from build123d import *

# Parameters (mm, degrees)
F0_R     = 11.5
F2_DEPTH = 2.3
F1_R     = 1.55
F3_DEPTH = 25
F4_R     = 1
F5_R     = 0.2


with BuildPart() as f2:
    # F0 (on Top) → F2 (new body)
    with BuildSketch(Plane.XY):
        Circle(F0_R)
    extrude(amount=F2_DEPTH)

    # F1 (on Top) → F3 (cut)
    with BuildSketch(Plane.XY):
        with Locations((0, -8.5)):
            Circle(F1_R)
    extrude(amount=F3_DEPTH, mode=Mode.SUBTRACT)

    # F4
    f4_edges = [f2.edges().sort_by_distance(p)[0] for p in [
        (-11.5, 0, 2.3),
        (-11.5, 0, 0),
    ]]
    fillet(f4_edges, radius=F4_R)

    # F5
    f5_edges = [f2.edges().sort_by_distance(p)[0] for p in [
        (-10.5, 0, 2.3),
        (-1.55, -8.5, 2.3),
        (-1.55, -8.5, 0),
    ]]
    fillet(f5_edges, radius=F5_R)


solid = f2.part
Verification items for the finished model (mm, model axes). Coordinates: 2 decimals unless noted, no trailing zeros. Loops run counter-clockwise (first coordinate to the right, second up) from the corner with the lowest first, then second, coordinate; pieces in that order, holes last. Notation, with made-up numbers: (-25.5, 26) -> (15.5, 26) arc R15 ccw to (15.5, 55) -> close; hole circle Ø8 at (-36, 3). An arc over 180 degrees is marked (long way). Answer as a JSON object with one key per item and string values. Group by question number.
Item 1: Sectioned sample at B-B on y = 0. Record the boundary of the cut face in (x, z).
Item 2: Sectioned sample at C-C on z = 0.5. Record the boundary of the cut face in (x, y).
Item 3: Sectioned sample at A-A on x = 0. Record the boundary of the cut face in (y, z), plus the area to 3 significant figures.
Item 4: Mould release check, pull along Y, two halves, no side actions. Record for faces 1 (the flat face through (0, 0, 0)), 2 (the cylindrical face through (-1.5, 11.4, 1.15)), 3 (the cylindrical face through (-0.336, -10.013, 1.137)): +Y half, -Y half, draft (parallel to the pull), parting line (faces both ways), or undercut.
Item 5: Scan lines: probe 1 along Y at (x, z) = (0, 1.35); probe 2 along X at (y, z) = (-8.5, 1.1); probe 3 along X at (y, z) = (-9, 0.95). Record each from-to range of solid material in increasing order.
Evaluation:
{
 "1": {"outline": "(-11.5, 1) arc R1 ccw to (-10.5, 0) -> (10.5, 0) arc R1 ccw to (11.5, 1) -> (11.5, 1.3) arc R1 ccw to (10.5, 2.3) -> (-10.5, 2.3) arc R1 ccw to (-11.5, 1.3) -> close"},
 "2": {"outline": "circle Ø22.73 at (0, 0); hole circle Ø3.1 at (0, -8.5)"},
 "3": {"outline": "(-11.5, 1) arc R1 ccw to (-10.5, 0) -> (-10.25, 0) arc R0.2 ccw to (-10.05, 0.2) -> (-10.05, 2.1) arc R0.2 ccw to (-10.25, 2.3) -> (-10.5, 2.3) arc R1 ccw to (-11.5, 1.3) -> close; (-6.95, 0.2) arc R0.2 ccw to (-6.75, 0) -> (10.5, 0) arc R1 ccw to (11.5, 1) -> (11.5, 1.3) arc R1 ccw to (10.5, 2.3) -> (-6.75, 2.3) arc R0.2 ccw to (-6.95, 2.1) -> close", "area": "44.9 mm²"},
 "4": {"face 1": "draft", "face 2": "parting line", "face 3": "undercut"},
 "5": {"probe 1": "y = -11.5 to -10.05, -6.95 to 11.5", "probe 2": "x = -7.75 to -1.55, 1.55 to 7.75", "probe 3": "x = -7.16 to -1.47, 1.47 to 7.16"}
}
